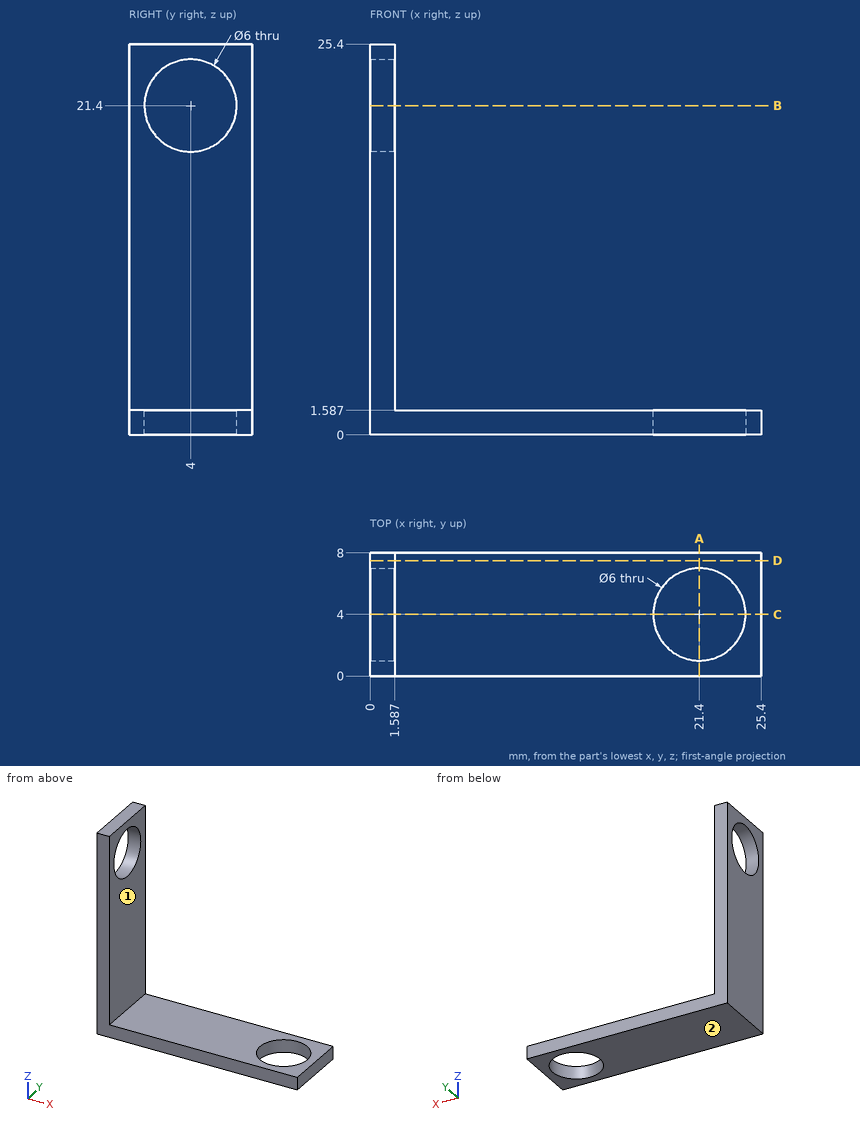
Source: three-view drawing plus pictorial views. Frame: mm from the lowest corner of the part. A direction names the side the tool comes from. Give positions to 0.01 mm unless a question says otherwise; leave off trailing zeros. Write each loop counter-clockwise with the first axis right and the second up, starting at its lowest first coordinate (ties: lowest second). Pieces come first, ordered by that corner, then holes. Notation, with made-up numbers: (32, 11) - (72, 11) arc R27 ccw to (72, 45) - close; hole circle Ø4 at (22.25, 41). An arc over 180 degrees is marked (long way). Write item = value, one per line. Start each with the question number.
Q1. Cut plane D-D, the plane y = 7.5. Return loops of the section in (x, z).
Q2. Material intervals for probe 1 along Y at (x, z) = (21.4, 1.2); probe 2 along X at (y, z) = (5.5, 14), sorted ascending.
Q3. Cut plane B-B, the plane z = 21.4. Return loops of the section in (x, y).
Q4. Cut plane C-C, the plane y = 4. Return loops of the section in (x, z).
Q5. Pin query (flat end, axial travel): pin 1 Ø2.5 at (y, z) = (5, 17) entering from +X; pin 2 Ø2.5 at (x, y) = (16, 6) entering from +Z. Return the tip coordinate at first contact, or that it passes through.
Q6. Reachability of the marked faces 1 and 2 from +Z, -Z, +X, -X, +Y, -Y: full face, straight path, thin tool, end or side. Return the list, or none.
Q7. Cut plane A-A, the plane x = 21.4. Return loops of the section in (y, z).
Computed values:
q1.outline = (0, 0) - (25.4, 0) - (25.4, 1.59) - (1.59, 1.59) - (1.59, 25.4) - (0, 25.4) - close
q2.probe_1 = 0 to 1, 7 to 8
q2.probe_2 = 0 to 1.59
q3.outline = (0, 0) - (1.59, 0) - (1.59, 1) - (0, 1) - close; (0, 7) - (1.59, 7) - (1.59, 8) - (0, 8) - close
q4.outline = (0, 0) - (18.4, 0) - (18.4, 1.59) - (1.59, 1.59) - (1.59, 18.4) - (0, 18.4) - close; (0, 24.4) - (1.59, 24.4) - (1.59, 25.4) - (0, 25.4) - close; (24.4, 0) - (25.4, 0) - (25.4, 1.59) - (24.4, 1.59) - close
q5.pin_1 = 1.59
q5.pin_2 = 1.59
q6.face_1 = +Z, +X, +Y, -Y
q6.face_2 = -Z, +X, -X, +Y, -Y
q7.outline = (0, 0) - (1, 0) - (1, 1.59) - (0, 1.59) - close; (7, 0) - (8, 0) - (8, 1.59) - (7, 1.59) - close
